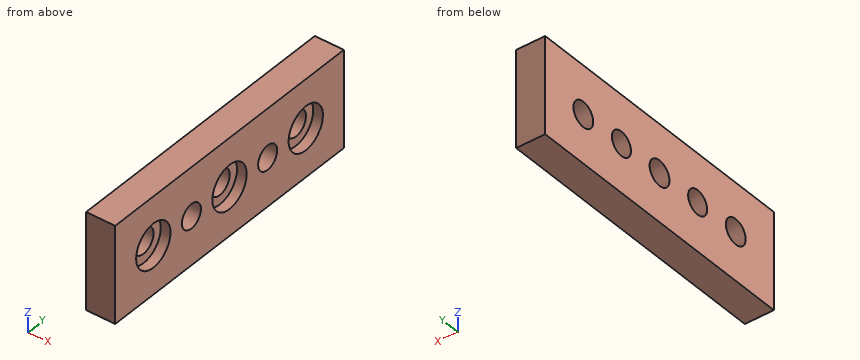
```python
from build123d import *

# Parameters (mm, degrees)
F0_W     = 60
F0_H     = 20
F0_R     = 2.6
F1_DEPTH = 6
F2_R     = 4.5
F3_DEPTH = 2
F4_R     = 2.5
F5_DEPTH = 25


with BuildPart() as f1:
    # F0 (on Right) → F1 (new body)
    with BuildSketch(Plane.YZ):
        Rectangle(F0_W, F0_H)
        with Locations((-20, 0)):
            Circle(F0_R, mode=Mode.SUBTRACT)
        Circle(F0_R, mode=Mode.SUBTRACT)
        with Locations((20, 0)):
            Circle(F0_R, mode=Mode.SUBTRACT)
    extrude(amount=F1_DEPTH)

    # F2 (on face) → F3 (cut)
    with BuildSketch(Plane.YZ.offset(6)):
        with Locations((-20, 0)):
            Circle(F2_R)
        Circle(F2_R)
        with Locations((20, 0)):
            Circle(F2_R)
    extrude(amount=-F3_DEPTH, mode=Mode.SUBTRACT)

    # F4 (on face) → F5 (cut)
    with BuildSketch(Plane.YZ.offset(6)):
        with Locations((-10, 0)):
            Circle(F4_R)
        with Locations((10, 0)):
            Circle(F4_R)
    extrude(amount=-F5_DEPTH, mode=Mode.SUBTRACT)


solid = f1.part
```
Part model, mm, in its own coordinate system. Coordinates: 2 decimals unless noted, no trailing zeros. Write each loop counter-clockwise with the first axis right and the second up, starting at its lowest first coordinate (ties: lowest second). Pieces come first, ordered by that corner, then holes.
Item 1: Pin check, flat tips, straight feed: pin 1 (3 mm diameter, centred on y = 0, z = 0, fed in from +X); pin 2 (7 mm diameter, centred on y = 20.5, z = -2, fed in from +X); pin 3 (4.5 mm diameter, centred on y = -20.5, z = -2, fed in from +X). Stop position of each tip, or through.
Item 2: Slice it at B-B (y = -20). Write the cut outline in (x, z).
Item 3: Slice it at C-C (z = 0). Count the separate pieces of the cut face and the enclosed holes in it, and give its area (3 significant figures).
Item 4: Probe line 1 (Z direction, x = 2, y = -20); line 2 (Z direction, x = 3.5, y = 10); line 3 (Y direction, x = 0.85, z = 1.5). List the from-to ranges inside material, lowest first.
Item 5: Slice it at D-D (y = 10). Write the cut outline in (x, z), and give its area (3 significant figures).
Item 6: Slice it at A-A (x = 5.15). Write the cut outline in (y, z), and give its area (3 significant figures).
Results found:
1. pin 1: passes through
1. pin 2: stops at x = 6
1. pin 3: stops at x = 4
2. outline: (0, -10) - (6, -10) - (6, -4.5) - (4, -4.5) - (4, -2.6) - (0, -2.6) - close; (0, 2.6) - (4, 2.6) - (4, 4.5) - (6, 4.5) - (6, 10) - (0, 10) - close
3. separate pieces: 6
3. enclosed holes: 0
3. area: 184 mm2
4. line 1: z = -10 to -2.6, 2.6 to 10
4. line 2: z = -10 to -2.5, 2.5 to 10
4. line 3: y = -30 to -22.12, -17.88 to -12, -8 to -2.12, 2.12 to 8, 12 to 17.88, 22.12 to 30
5. outline: (0, -10) - (6, -10) - (6, -2.5) - (0, -2.5) - close; (0, 2.5) - (6, 2.5) - (6, 10) - (0, 10) - close
5. area: 90.0 mm2
6. outline: (-30, -10) - (30, -10) - (30, 10) - (-30, 10) - close; hole circle Ø9 at (-20, 0); hole circle Ø5 at (-10, 0); hole circle Ø9 at (0, 0); hole circle Ø5 at (10, 0); hole circle Ø9 at (20, 0)
6. area: 970 mm2
